Part print with two shaded views. Sizes in mm from the minimum x, y, z corner. A direction names the side the tool comes from. Give positions to 0.01 mm unless a question says otherwise; leave off trailing zeros. Loops run counter-clockwise (first coordinate to the right, second up) from the corner with the lowest first, then second, coordinate; pieces in that order, holes last. Notation, with made-up numbers: M 4,40.25 L 17,40.25 A17 cw 17,71.25 Z; hole C -2.5,22.25 d1. An arc over 180 degrees is marked long. Answer in a Markdown table with one row per item.
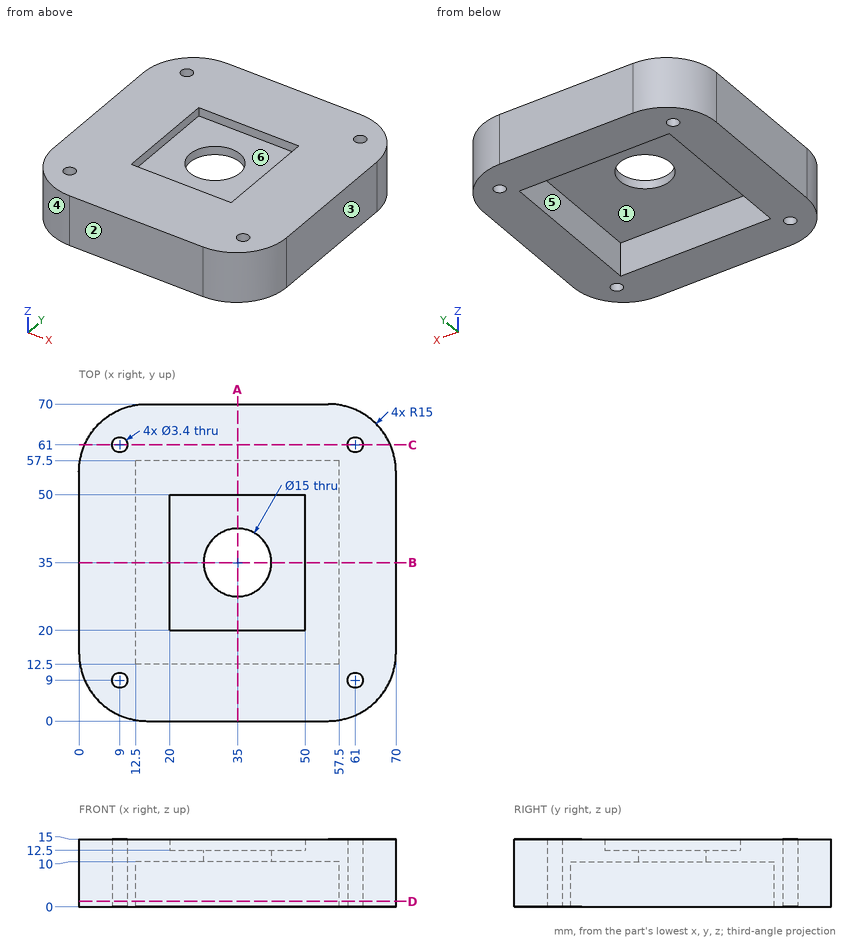
Q1. 3-axis set-ups, long thin cutter, end or side, ignore diameter. For the marked faces 4, 5 and 6: which of +Z, -Z, +X, -X, +Y, -Y reach the whole face in a straight line?
Reported:
| item | result |
|---|---|
| face 4 | +Z, -Z, -X, -Y |
| face 5 | -Z |
| face 6 | +Z |
Q2. Saw through at C-C (y = 61). Give the cut face in (x, z), and give its area (3 significant figures).
Reported:
| item | result |
|---|---|
| outline | M 1.25,0 L 7.3,0 L 7.3,15 L 1.25,15 Z; M 10.7,0 L 59.3,0 L 59.3,15 L 10.7,15 Z; M 62.7,0 L 68.75,0 L 68.75,15 L 62.7,15 Z |
| area | 910 mm² |
Q3. Probe probe 1 along Y at (x, z) = (39, 13.25); probe 2 along X at (y, z) = (30, 6); probe 3 along Y at (x, z) = (61, 6.5). List the from-to ranges inside material, lowest first.
Reported:
| item | result |
|---|---|
| probe 1 | 0 to 20, 50 to 70 |
| probe 2 | 0 to 12.5, 57.5 to 70 |
| probe 3 | 1.25 to 7.3, 10.7 to 59.3, 62.7 to 68.75 |
Q4. Saw through at A-A (x = 35). Give the cut face in (y, z), and give its area (4 significant figures).
Reported:
| item | result |
|---|---|
| outline | M 0,0 L 12.5,0 L 12.5,10 L 27.5,10 L 27.5,12.5 L 20,12.5 L 20,15 L 0,15 Z; M 42.5,10 L 57.5,10 L 57.5,0 L 70,0 L 70,15 L 50,15 L 50,12.5 L 42.5,12.5 Z |
| area | 487.5 mm² |
Q5. Drop flat-ended pins along their axis: pin 1 (5 mm diameter, centred on y = 8, z = 10.5, fed in from +X); pin 2 (17 mm diameter, centred on x = 35, y = 35, fed in from +Z). Give the stop position or say it passes through.
Reported:
| item | result |
|---|---|
| pin 1 | x = 69.31 |
| pin 2 | z = 12.5 |
Q6. Mould opens along X. For the marked faces 1, 2 and 3 say: released by +X, released by -X, zero draft, split by the parting line, or undercut.
Reported:
| item | result |
|---|---|
| face 1 | undercut |
| face 2 | zero draft |
| face 3 | released by +X |
Q7. Saw through at D-D (z = 1.25). Give the cut face in (x, y).
Reported:
| item | result |
|---|---|
| outline | M 0,15 A15 ccw 15,0 L 55,0 A15 ccw 70,15 L 70,55 A15 ccw 55,70 L 15,70 A15 ccw 0,55 Z; hole C 9,9 d3.4; hole C 9,61 d3.4; hole M 12.5,12.5 L 57.5,12.5 L 57.5,57.5 L 12.5,57.5 Z; hole C 61,9 d3.4; hole C 61,61 d3.4 |
